Answer from the drawing. Dimensions are ordinates in mm from the lowest x, y and z of the part. A direction names the side the tool comes from. Round coordinates to 2 decimals unless told otherwise and drop trailing zeros. Order: outer loops, then holes, each group sorted by start corner. A loop starts at its lowest first (then second) coordinate and runs counter-clockwise, first axis right, second up. Notation, with made-up numbers: (-24, 23.5) -> (-2, 23.5) arc R24 cw to (-2, 58.5) -> close; hole circle Ø8 at (27.25, 4). An arc over 180 degrees is marked (long way). Use a Markdown table: item, result. Add a question column.
Item 1: A cutting plane is placed at B-B, the plane x = 5. Determine the outline of the cut face in (y, z), plus the area to 3 significant figures.
Item 2: A tool of negligible diameter and unlimited length cuts with its end or side. For the marked faces 1, 2 and 3, from which of +Z, -Z, +X, -X, +Y, -Y can it reach the whole face along a straight path? Write none if from no direction.
Item 3: Find the intervals of material crossed by L1, parallel to X at y = 1.05, z = 5; L2, parallel to Y at x = 32, z = 44.5; L3, parallel to X at y = 3.5, z = 47, in increasing order. Write a range as [from, to].
Item 4: Flat-ended cylindrical pins translate along their axes: P1, Ø4.5, axis at x = 5, z = 5, coming from the +Y side; P2, Ø4, axis at y = 5.5, z = 22.5, coming from the +X side; P3, Ø4, axis at y = 6.5, z = 16.5, coming from the -X side. Find the tip coordinate at first contact, or state that the pin passes through.
Item 5: A cutting plane is placed at C-C, the plane z = 8. Determine the outline of the cut face in (x, y).
Item 6: A cutting plane is placed at A-A, the plane z = 47. Determine the outline of the cut face in (x, y).
Item 7: A cutting plane is placed at D-D, the plane y = 7. Determine the outline of the cut face in (x, z), plus the area to 3 significant figures.
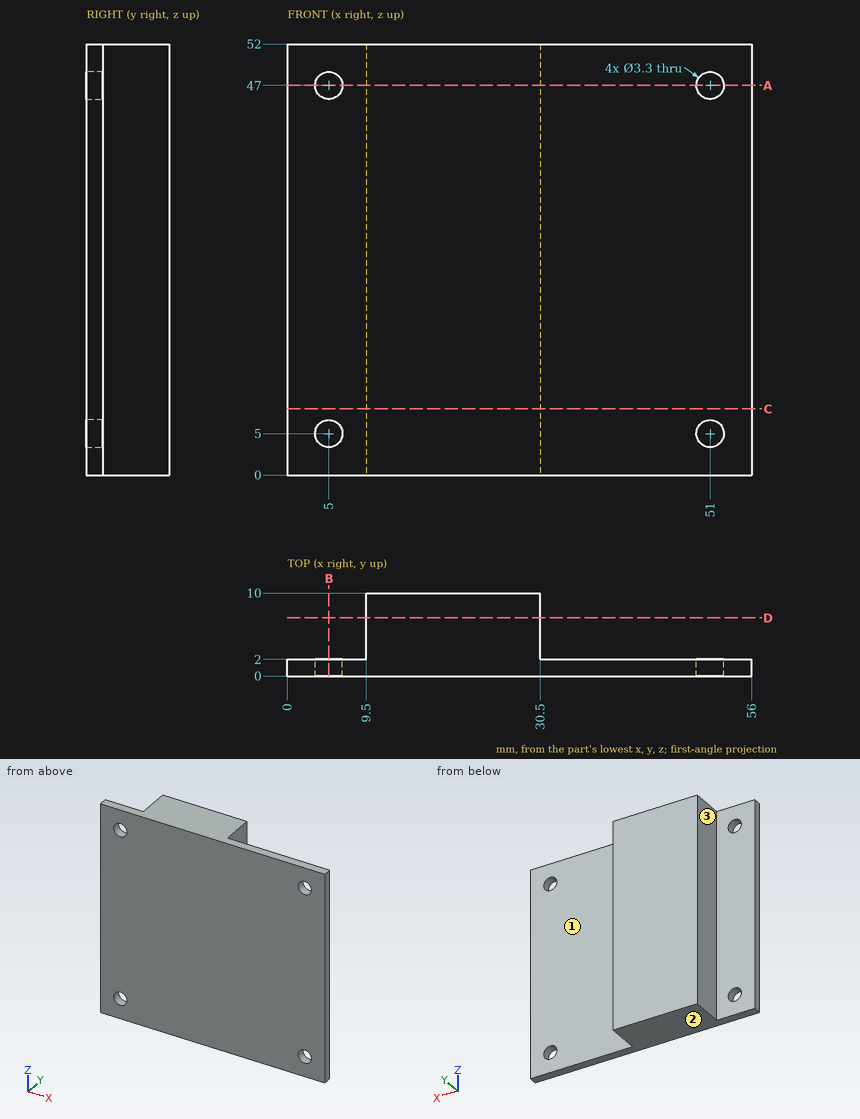
Reported:
| question | item | result |
|---|---|---|
| 1 | outline | (0, 0) -> (2, 0) -> (2, 3.35) -> (0, 3.35) -> close; (0, 6.65) -> (2, 6.65) -> (2, 45.35) -> (0, 45.35) -> close; (0, 48.65) -> (2, 48.65) -> (2, 52) -> (0, 52) -> close |
| 1 | area | 90.8 mm² |
| 2 | face 1 | +Z, -Z, +X, +Y |
| 2 | face 2 | -Z, +X, -X, +Y, -Y |
| 2 | face 3 | +Z, -Z, -X, +Y |
| 3 | L1 | [0, 3.35], [6.65, 49.35], [52.65, 56] |
| 3 | L2 | [0, 2] |
| 3 | L3 | [9.5, 30.5] |
| 4 | P1 | y = 2 |
| 4 | P2 | x = 30.5 |
| 4 | P3 | x = 9.5 |
| 5 | outline | (0, 0) -> (56, 0) -> (56, 2) -> (30.5, 2) -> (30.5, 10) -> (9.5, 10) -> (9.5, 2) -> (0, 2) -> close |
| 6 | outline | (0, 0) -> (3.35, 0) -> (3.35, 2) -> (0, 2) -> close; (6.65, 0) -> (49.35, 0) -> (49.35, 2) -> (30.5, 2) -> (30.5, 10) -> (9.5, 10) -> (9.5, 2) -> (6.65, 2) -> close; (52.65, 0) -> (56, 0) -> (56, 2) -> (52.65, 2) -> close |
| 7 | outline | (9.5, 0) -> (30.5, 0) -> (30.5, 52) -> (9.5, 52) -> close |
| 7 | area | 1,090 mm² |
